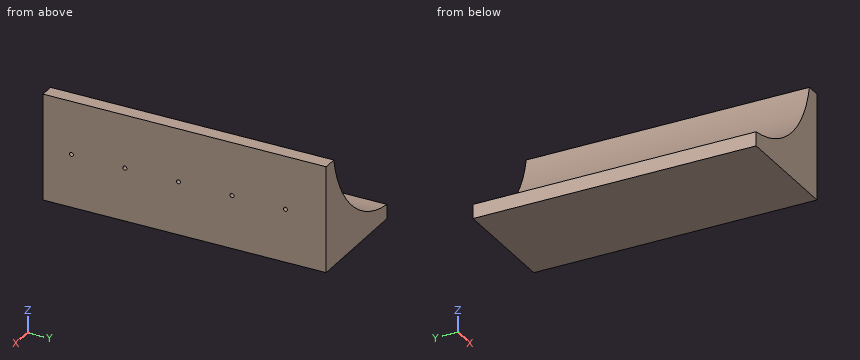
from build123d import *

# Parameters (mm, degrees)
F1_DEPTH = 254
F3_D     = 3.5814
F3_DEPTH = 19.05
F3_TIP   = 1.0759611105


with BuildPart() as f1:
    # F0 (on Front) → F1 (new body)
    with BuildSketch(Plane.XZ):
        Polygon((49.1248931152, -56.7675527828), (-39.7751068848, -57.0361235134), (48.4362465841, -57.0361235134), (49.1248931152, -57.0361235134), align=None)
        with BuildLine():
            ThreePointArc((49.1248931152, 25.5138764866), (18.3482789064, -30.4863082116), (-39.7751068848, -57.0361235134))
            Line((-39.7751068848, -57.0361235134), (49.1248931152, -56.7675527828))
            Line((49.1248931152, -56.7675527828), (49.1248931152, 25.5138764866))
        make_face()
        Polygon((48.4362465841, -57.0361235134), (-39.7751068848, -57.0361235134), (-39.7751068848, -69.7361235134), (61.8248931152, -69.7361235134), (61.8248931152, -57.0361235134), (55.4748931152, -57.0361235134), (49.1248931152, -57.0361235134), align=None)
        Polygon((49.1248931152, 25.5138764866), (49.1248931152, -56.7675527828), (49.1248931152, -57.0361235134), (55.4748931152, -57.0361235134), (61.8248931152, -57.0361235134), (61.8248931152, 25.5138764866), align=None)
    extrude(amount=F1_DEPTH)

    # F3
    with Locations(Plane.YZ.offset(61.8248931152)):
        with Locations((-228.5564392805, -22.1111235134), (-180.5504392805, -22.1111235134), (-132.5444392805, -22.1111235134), (-84.5384392805, -22.1111235134), (-36.5324392805, -22.1111235134)):
            Hole(F3_D / 2, depth=F3_DEPTH)
            with Locations((0, 0, -(F3_DEPTH + F3_TIP / 2))):  # 118° drill point
                Cone(0, F3_D / 2, F3_TIP, mode=Mode.SUBTRACT)


solid = f1.part
Here's how the part is built. I have some questions about the finished solid (model axes, mm). Coordinates: 2 decimals unless noted, no trailing zeros. Order: outer loops, then holes, each group sorted by start corner. A loop starts at its lowest first (then second) coordinate and runs counter-clockwise, first axis right, second up. Notation, with made-up numbers: M 78,-18.75 L 84,-18.75 A18 cw 84,-7.75 Z; hole C 30.5,49.25 d3. An arc over 180 degrees is marked long. Answer as CSV lines item,"result".
Item 1: Imagine slicing it at B-B on z = -53. Write out the boundary of the cut face in (x, y).
Results found:
outline,"M -20.45,-254 L 61.82,-254 L 61.82,0 L -20.45,0 Z"
Item 2: Imagine slicing it at C-C on x = 19. Write out the boundary of the cut face in (y, z).
Results found:
outline,"M -254,-69.74 L 0,-69.74 L 0,-29.88 L -254,-29.88 Z"
Item 3: If I drill on line 1 (X direction, y = -79, z = -15); line 2 (X direction, y = -31.5, z = -42); line 3 (Z direction, x = 40, y = -172), over which ranges is the centre line in solid material (lowest first)?
Results found:
line 1,"31.95 to 61.82"
line 2,"3.37 to 61.82"
line 3,"-69.74 to -1.65"
Item 4: For pin 1 (4 mm diameter, centred on x = 12.5, y = -145.5, fed in from +Z); pin 2 (4 mm diameter, centred on y = -36.53, z = -22.11, fed in from -X); pin 3 (5.5 mm diameter, centred on y = -180.55, z = -22.11, fed in from -X), each with a flat end and sliding along its axis, tell me the tip position at first contact or that it passes through.
Results found:
pin 1,"z = -33.88"
pin 2,"x = 24.64"
pin 3,"x = 23.95"
Item 5: Imagine slicing it at A-A on y = -153. Write out the boundary of the cut face in (x, z).
Results found:
outline,"M -39.78,-69.74 L 61.82,-69.74 L 61.82,25.51 L 49.12,25.51 A101.6 cw -39.78,-57.04 Z"
